Could you check a few things on this model? Use its own coordinates, in mm. A direction names the side the tool comes from. Give positions to 0.01 mm unless a question says otherwise; leave off trailing zeros. Loops run counter-clockwise (first coordinate to the right, second up) from the corner with the lowest first, then second, coordinate; pieces in that order, holes last. Notation, with made-up numbers: (15, 19) -> (22, 19) arc R20 cw to (22, 24) -> close; hole circle Ø11 at (11, -23.5). An arc over 180 degrees is marked (long way). Write each question's results on one line, items separated by ' | '. Start each with the question number.
Q1. Which directions (+Z, -Z, +X, -X, +Y, -Y) give clear straight access to the entire face, cutting with the end or side of a thin tool? Please do faces 5 (the face through (6.6, 1.6, 57.6)), 6 (the face through (5.08, -1, -22)).
Q2. We'd pull the mould along Y, two halves only. Please class faces 1 (the face through (3.32, -18.78, 0.95)), 2 (the face through (6, 38.1, 14)), 3 (the face through (8.837, -9.336, 11.275)), 4 (the face through (6.876, 1.576, 0.166)): released by +Y, released by -Y, zero draft, split by the parting line, or undercut.
Q3. Will these pins go through, and if not, where does the flat tip stop? P1, Ø12.5, axis at y = 0, z = 38.1, coming from the -X side; P2, Ø4, axis at x = 6.35, z = 57.15, coming from the -Y side; P3, Ø8, axis at y = -11, z = 11, coming from the -X side; P4, Ø5, axis at x = 6.35, z = 0, coming from the -Y side.
Q4. If we section it at A-A, the plane z = 38.1: List the corners of the cut face in (x, y) for me.
Q5. If I drill on line 1 along Z through (x, y) = (6.35, -22) (3 decimals); line 2 along Z through (x, y) = (9.75, -11); line 3 along X through (y, z) = (-11, 0) (3 decimals), over which ranges is the centre line in solid material (lowest first)?
from build123d import *

# Parameters (mm, degrees)
SKETCH1_R                       = 3.854557775
SKETCH1_W                       = 25.4
SKETCH1_H                       = 76.2
BOSS_EXTRUDE1_DEPTH             = 12.7
F_1_4_0_25_DIAMETER_HOLE2_D     = 6.35
F_1_4_0_25_DIAMETER_HOLE2_DEPTH = 38.1
F_1_4_0_25_DIAMETER_HOLE2_TIP   = 1.907732465
SKETCH2_R                       = 7.9375
CUT_EXTRUDE1_DEPTH              = 5.08


with BuildPart() as part:
    # Sketch1 → Boss-Extrude1 (new body)
    # profile 1 of 3: a face of its own
    with BuildSketch(Plane(origin=(0, 0, 0), x_dir=(0, 0, -1), z_dir=(1, 0, 0))):
        with BuildLine():
            Line((-76.2, 38.1), (-76.2, 0))
            Line((-76.2, 0), (-41.954557775, 0))
            ThreePointArc((-41.954557775, 0), (-38.1, 3.854557775), (-34.245442225, 0))
            Line((-34.245442225, 0), (14.762299925, 0))
            ThreePointArc((14.762299925, 0), (17.903949731, 4.910646748), (22.312291357, 1.096077429))
            ThreePointArc((22.312291357, 1.096077429), (22.272302901, 0.542293578), (22.153167239, 0))
            Line((22.153167239, 0), (76.2, 0))
            Line((76.2, 0), (76.2, 38.1))
            Line((76.2, 38.1), (-76.2, 38.1))
        make_face()
    # profile 2 of 3: a face of its own
    with BuildSketch(Plane(origin=(0, 0, 0), x_dir=(0, 0, -1), z_dir=(1, 0, 0))):
        with BuildLine():
            Line((-41.954557775, 0), (-76.2, 0))
            Line((-76.2, 0), (-76.2, -38.1))
            Line((-76.2, -38.1), (76.2, -38.1))
            Line((76.2, -38.1), (76.2, 0))
            Line((76.2, 0), (22.153167239, 0))
            ThreePointArc((22.153167239, 0), (18.457733582, -2.758480346), (14.762299925, 0))
            Line((14.762299925, 0), (-34.245442225, 0))
            ThreePointArc((-34.245442225, 0), (-38.1, -3.854557775), (-41.954557775, 0))
        make_face()
        with Locations((-14.836022013, -7.860160654)):
            Circle(SKETCH1_R, mode=Mode.SUBTRACT)
        with Locations((51.143457994, -9.873506971)):
            Circle(SKETCH1_R, mode=Mode.SUBTRACT)
    # profile 3 of 3: a face of its own
    with BuildSketch(Plane(origin=(0, 0, 0), x_dir=(0, 0, -1), z_dir=(1, 0, 0))):
        with Locations((-88.9, 0)):
            Rectangle(SKETCH1_W, SKETCH1_H)
    extrude(amount=BOSS_EXTRUDE1_DEPTH)

    # 1_4 _0.25_ Diameter Hole2
    with Locations(Plane.XZ.offset(38.1)):
        with Locations((6.35, 57.15), (6.35, -63.5), (6.35, 0)):
            Hole(F_1_4_0_25_DIAMETER_HOLE2_D / 2, depth=F_1_4_0_25_DIAMETER_HOLE2_DEPTH)
            with Locations((0, 0, -(F_1_4_0_25_DIAMETER_HOLE2_DEPTH + F_1_4_0_25_DIAMETER_HOLE2_TIP / 2))):  # 118° drill point
                Cone(0, F_1_4_0_25_DIAMETER_HOLE2_D / 2, F_1_4_0_25_DIAMETER_HOLE2_TIP, mode=Mode.SUBTRACT)

    # Sketch2 → Cut-Extrude1 (cut)
    with BuildSketch(Plane.ZY):
        with Locations((38.1, 0)):
            Circle(SKETCH2_R)
        with Locations((14.836022013, -7.860160654)):
            Circle(SKETCH2_R)
        with Locations((-18.457733582, 1.096077429)):
            Circle(SKETCH2_R)
        with Locations((-51.143457994, -9.873506971)):
            Circle(SKETCH2_R)
    extrude(amount=-CUT_EXTRUDE1_DEPTH, mode=Mode.SUBTRACT)


solid = part.part
Final values:
1) face 5: -Y | face 6: -X
2) face 1: zero draft | face 2: released by +Y | face 3: undercut | face 4: released by -Y
3) P1: stops at x = 5.08 | P2: stops at y = 0.71 | P3: stops at x = 0 | P4: stops at y = 0.41
4) outline: (0, -38.1) -> (12.7, -38.1) -> (12.7, -3.85) -> (5.08, -3.85) -> (5.08, -7.94) -> (0, -7.94) -> close; (0, 7.94) -> (5.08, 7.94) -> (5.08, 3.85) -> (12.7, 3.85) -> (12.7, 38.1) -> (0, 38.1) -> close
5) line 1: z = -76.2 to -66.675, -60.325 to -3.175, 3.175 to 53.975, 60.325 to 101.6 | line 2: z = -76.2 to -54.83, -47.46 to 12.6, 17.07 to 101.6 | line 3: x = 0 to 3.175, 9.525 to 12.7
